```python
from build123d import *

# Parameters (mm, degrees)
F0_R     = 22.2885
F1_DEPTH = 6.35


with BuildPart() as f1:
    # F0 (on Top) → F1 (new body)
    with BuildSketch(Plane.XY):
        with BuildLine():
            Line((-33.337868, -24.8285), (0, -24.8285))
            ThreePointArc((0, -24.8285), (24.8285, 0), (0, 24.8285))
            Line((0, 24.8285), (-39.6875, 24.8285))
            Line((-39.6875, 24.8285), (-39.6875, -86.2965))
            Line((-39.6875, -86.2965), (-33.337868, -86.228111))
            Line((-33.337868, -86.228111), (-33.337868, -24.8285))
        make_face()
        Circle(F0_R, mode=Mode.SUBTRACT)
    extrude(amount=F1_DEPTH)


solid = f1.part
```
Read the model definition and answer for the solid it produces. Units are mm, in the model's axes. A direction names the side the tool comes from. Give positions to 0.01 mm unless a question says otherwise; leave off trailing zeros. Order: outer loops, then holes, each group sorted by start corner. A loop starts at its lowest first (then second) coordinate and runs counter-clockwise, first axis right, second up.
(1) For faces 1 (the flat face through (-39.688, -30, 3)), 2 (the flat face through (-17, -24.828, 3)), determine the directions among +Z, -Z, +X, -X, +Y, -Y from which every point of the face is accessible in a straight line to the end or side of a thin tool.
(2) Find section B-B (z = 5). Give the vertices of the cut face in (x, y).
(3) Find section A-A (y = 0). Give the vertices of the cut face in (x, z), plus the area to 3 significant figures.
(4) Find section C-C (x = 4.5). Give the vertices of the cut face in (y, z), plus the area to 3 significant figures.
(5) For a pull along Y with two mould halves and no side action, classify faces 3 (the cylindrical face through (24.822, -0.546, 3.131)), 4 (the flat face through (-24, -14, 0)), 5 (the cylindrical face through (-2.9, 22.1, 3.1)), 6 (the flat face through (-20, 24.828, 3)) as released by +Y, released by -Y, zero draft, split by the parting line, or undercut.
(6) Given pin 1 (1.9 mm diameter, centred on y = -50.5, z = 4.5, fed in from +X), flat-ended and moving along its own axis, determine where the tip first touches the part or whether it passes through.
(7) Find section D-D (y = -33.5). Give the vertices of the cut face in (x, z).
(8) Straight lines are drawn through the part: L1, parallel to Y at x = -31, z = 4; L2, parallel to X at y = -78, z = 0.75; L3, parallel to Y at x = 4, z = 1.5. For each, find the intervals that lie inside material, in ascending order.
Result sheet:
1. face 1: +Z, -Z, -X, +Y, -Y
1. face 2: +Z, -Z, +X, -Y
2. outline: (-39.69, -86.3) - (-33.34, -86.23) - (-33.34, -24.83) - (0, -24.83) arc R24.83 ccw to (0, 24.83) - (-39.69, 24.83) - close; hole circle Ø44.58 at (0, 0)
3. outline: (-39.69, 0) - (-22.29, 0) - (-22.29, 6.35) - (-39.69, 6.35) - close; (22.29, 0) - (24.83, 0) - (24.83, 6.35) - (22.29, 6.35) - close
3. area: 127 mm2
4. outline: (-24.42, 0) - (-21.83, 0) - (-21.83, 6.35) - (-24.42, 6.35) - close; (21.83, 0) - (24.42, 0) - (24.42, 6.35) - (21.83, 6.35) - close
4. area: 32.9 mm2
5. face 3: split by the parting line
5. face 4: zero draft
5. face 5: undercut
5. face 6: released by +Y
6. pin 1: stops at x = -33.34
7. outline: (-39.69, 0) - (-33.34, 0) - (-33.34, 6.35) - (-39.69, 6.35) - close
8. L1: y = -24.83 to 24.83
8. L2: x = -39.69 to -33.34
8. L3: y = -24.5 to -21.93, 21.93 to 24.5
